Part model, mm, in its own coordinate system. A direction names the side the tool comes from. Coordinates: 2 decimals unless noted, no trailing zeros. Loops run counter-clockwise (first coordinate to the right, second up) from the corner with the lowest first, then second, coordinate; pieces in that order, holes last. Notation, with made-up numbers: (23, 67) -> (47, 67) arc R24 ccw to (47, 89) -> close; hole circle Ø10 at (49.5, 84). An arc over 180 degrees is marked (long way). One line per question, with ' | ' between items. Start each with the question number.
1) Cut at A-A (y = -4.5). List the corners of the cut face in (x, z).
2) 3-axis set-ups, long thin cutter, end or side, ignore diameter. For faces 4 (the face through (79, -4, -1.2)), 5 (the face through (160, -1, -4)): which of +Z, -Z, +X, -X, +Y, -Y reach the whole face in a straight line?
3) Two-plate mould, pull along Y, no slides. Class faces 1 (the face through (79, -9, -4)), 2 (the face through (79, -5, -9)), 3 (the face through (4.05, -5.93, -8.41)): released by +Y, released by -Y, zero draft, split by the parting line, or undercut.
4) Cut at C-C (z = -4.5). List the corners of the cut face in (x, y).
5) Cut at D-D (x = 4.5). List the corners of the cut face in (y, z), plus the area to 3 significant figures.
6) Cut at B-B (x = 83). List the corners of the cut face in (y, z), plus the area to 3 significant figures.
7) Probe L1, parallel to X at y = -8.45, z = -4.5; L2, parallel to Z at x = 35, y = -1.5. List the from-to ranges inside material, lowest first. Write a range as from..to.
8) Drop a flat-ended pin along its axis: pin 1 (3.5 mm diameter, centred on x = 156.5, z = -4.5, fed in from +Y). Give the stop position or say it passes through.
Autodesk Inventor part; units mm, degrees
ref_plane "YZ Plane" through (0, 0, 0) normal (1, 0, 0) x (0, 1, 0)
ref_plane "XZ Plane" through (0, 0, 0) normal (0, 1, 0) x (-1, 0, 0)
ref_plane "XY Plane" through (0, 0, 0) normal (0, 0, 1) x (1, 0, 0)
sketch "スケッチ1" plane through (0, 0, 0) normal (1, 0, 0) x (0, 1, 0)
  line L0 (0, 0) -> (-9, 0)
  line L1 (-9, 0) -> (-9, -9)
  line L2 (-9, -9) -> (0, -9)
  line L3 (0, -9) -> (0, 0)
  line L4 (-1.2, -1.2) -> (-7.8, -1.2)
  line L5 (-7.8, -1.2) -> (-7.8, -7.8)
  line L6 (-7.8, -7.8) -> (-1.2, -7.8)
  line L7 (-1.2, -7.8) -> (-1.2, -1.2)
  dimension "d0" = 9
  dimension "d1" = 9
  dimension "d2" = 6.6
  dimension "d3" = 6.6
  dimension "d4" = 1.2
  dimension "d5" = 1.2
extrude "押し出し1" add sketch "スケッチ1" along normal blind 160
sketch "スケッチ2" plane through (0, 0, 0) normal (0, 1, 0) x (1, 0, 0)
  line L0 (0, 9) -> (160, 9)
  line L1 (0, 9) -> (0, 0)
  line L2 (160, 9) -> (160, 0)
  point P0 (13.5, 4.5)
  point P1 (156.5, 4.5)
  dimension "d8" = 4.5
  dimension "d9" = 4.5
  dimension "d10" = 13.5
  dimension "d11" = 3.5
hole "穴1" at (13.5, 0, -4.5) at (156.5, 0, -4.5) direction (0, -1, 0) diameter 3 end through all
sketch "スケッチ3" plane through (0, -9, 0) normal (0, 0, 1) x (1, 0, 0)
  line L0 (0, 9) -> (160, 9)
  line L1 (0, 9) -> (0, 0)
  point P0 (4.5, 4.5)
  dimension "d19" = 4.5
  dimension "d20" = 4.5
hole "穴2" at (4.5, -4.5, 0) direction (0, 0, -1) diameter 3 end through all
equation "\"d3\" = d2"
equation "\"d5\" = d4"
properties part number "ハンド9x9_6" material "アルミニウム 6061"
Reported:
1) outline: (0, -9) -> (3, -9) -> (3, -7.8) -> (0, -7.8) -> close; (0, -1.2) -> (3, -1.2) -> (3, 0) -> (0, 0) -> close; (6, -9) -> (160, -9) -> (160, -7.8) -> (6, -7.8) -> close; (6, -1.2) -> (160, -1.2) -> (160, 0) -> (6, 0) -> close
2) face 4: +X, -X | face 5: +Z, -Z, +X, +Y, -Y
3) face 1: released by -Y | face 2: zero draft | face 3: undercut
4) outline: (0, -9) -> (12, -9) -> (12, -7.8) -> (0, -7.8) -> close; (0, -1.2) -> (12, -1.2) -> (12, 0) -> (0, 0) -> close; (15, -9) -> (155, -9) -> (155, -7.8) -> (15, -7.8) -> close; (15, -1.2) -> (155, -1.2) -> (155, 0) -> (15, 0) -> close; (158, -9) -> (160, -9) -> (160, -7.8) -> (158, -7.8) -> close; (158, -1.2) -> (160, -1.2) -> (160, 0) -> (158, 0) -> close
5) outline: (-9, -9) -> (-6, -9) -> (-6, -7.8) -> (-7.8, -7.8) -> (-7.8, -1.2) -> (-6, -1.2) -> (-6, 0) -> (-9, 0) -> close; (-3, -9) -> (0, -9) -> (0, 0) -> (-3, 0) -> (-3, -1.2) -> (-1.2, -1.2) -> (-1.2, -7.8) -> (-3, -7.8) -> close | area: 30.2 mm²
6) outline: (-9, -9) -> (0, -9) -> (0, 0) -> (-9, 0) -> close; hole (-7.8, -7.8) -> (-1.2, -7.8) -> (-1.2, -1.2) -> (-7.8, -1.2) -> close | area: 37.4 mm²
7) L1: x = 0..12, 15..155, 158..160 | L2: z = -9..-7.8, -1.2..0
8) pin 1: stops at y = 0
